Can you work these out from the model? Positions are in its coordinate system, mm. Coordinates: 2 decimals unless noted, no trailing zeros. Loops run counter-clockwise (first coordinate to the right, second up) from the corner with the lowest first, then second, coordinate; pieces in that order, holes last. Notation, with made-up numbers: (52.25, 26) -> (69.25, 26) arc R27 cw to (69.25, 56) -> close; hole circle Ø4 at (55, 74.5). An arc over 180 degrees is marked (long way). Put each result on its own line as item: value. Start each with the question number.
Item 1: Please list where these lines run through material, in increasing order: L1, parallel to Y at x = 298.65, z = 25.27; L2, parallel to X at y = 3, z = 12; L3, parallel to X at y = 31.5, z = 26. Write a range as from..to.
Item 2: If we section it at A-A on x = 29.5: Please give me the cut outline in (y, z), plus the area to 3 significant figures.
Item 3: Will these pins go through, and if not, where does the flat tip stop? P1, Ø6, axis at x = 187, z = 31, coming from the +Y side; P2, Ø5, axis at x = 217.5, z = 27.5, coming from the +Y side; P3, Ø3.5, axis at y = 27.39, z = 25.27, coming from the +X side.
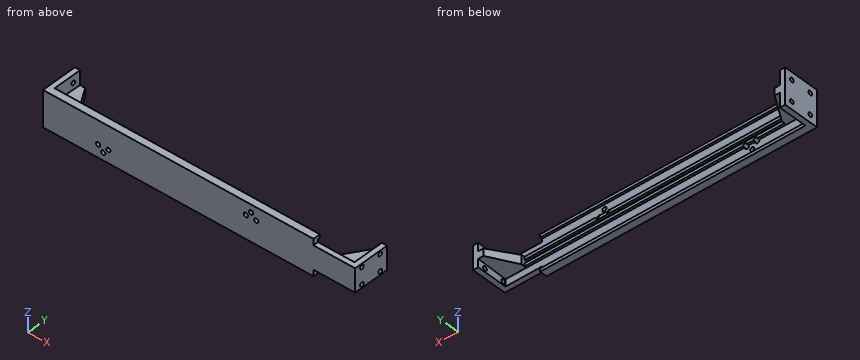
```python
from build123d import *

# Parameters (mm, degrees)
EXTRUDE_1_DEPTH          = 34.54
CUT_EXTRUDE_1_REACH      = 305.978
SKETCH_2_W               = 40
SKETCH_2_H               = 6
SKETCH_3_R               = 2
CUT_EXTRUDE_2_DEPTH      = 5
SKETCH_4_R               = 2
CUT_EXTRUDE_3_DEPTH      = 5
RIB_START                = 5
RIB_7_DEPTH              = 20
RIB_START_2              = 12.730059485
RIB_7_2_DEPTH            = 9.07988103
RIB_START_3              = 275
RIB_19_DEPTH             = 20
RIB_START_4              = 147.269934089
RIB_19_2_DEPTH           = 35.576868781
EXTRUDE_2_REACH          = 301.045
SKETCH_8_W               = 3
SKETCH_8_H               = 2
CUT_EXTRUDE_4_DEPTH      = 304.978058419
CUT_EXTRUDE_4_DEPTH_BACK = 304.978058419
SKETCH_9_W               = 35
SKETCH_9_H               = 3
CUT_EXTRUDE_5_REACH      = 305.978
SKETCH_10_R              = 2
CUT_EXTRUDE_6_REACH      = 305.978
SKETCH_11_R              = 2


with BuildPart() as part:
    # 草图1 → 凸台-拉伸1 (new body)
    with BuildSketch(Plane.XY):
        Polygon((0, 0), (300, 0), (300, 34.78), (295, 34.78), (295, 5), (5, 5), (5, 34.78), (0, 34.78), align=None)
    extrude(amount=EXTRUDE_1_DEPTH)

    # 切除-拉伸1: up to this face of the body (flat: up to its plane)
    cut_extrude_1_end = Plane(part.part.faces().sort_by_distance((297.5, 34.78, 17.27))[0])
    # 草图2 → 切除-拉伸1 (cut, up to the picked face)
    with BuildSketch(Plane.XZ, mode=Mode.PRIVATE) as cut_extrude_1_sk1:
        with Locations((280, 31.54)):
            Rectangle(SKETCH_2_W, SKETCH_2_H)
    cut_extrude_1_tool1 = split(extrude(cut_extrude_1_sk1.sketch, amount=-CUT_EXTRUDE_1_REACH, mode=Mode.PRIVATE), bisect_by=cut_extrude_1_end, keep=Keep.BOTH, mode=Mode.PRIVATE)
    # 草图2 → 切除-拉伸1 (cut, up to the picked face)
    with BuildSketch(Plane.XZ, mode=Mode.PRIVATE) as cut_extrude_1_sk2:
        with Locations((280, 3)):
            Rectangle(SKETCH_2_W, SKETCH_2_H)
    cut_extrude_1_tool2 = split(extrude(cut_extrude_1_sk2.sketch, amount=-CUT_EXTRUDE_1_REACH, mode=Mode.PRIVATE), bisect_by=cut_extrude_1_end, keep=Keep.BOTH, mode=Mode.PRIVATE)
    add(cut_extrude_1_tool1.solids().sort_by(Axis((280, 0, 31.54), (0, 1, 0)))[0], mode=Mode.SUBTRACT)
    add(cut_extrude_1_tool2.solids().sort_by(Axis((280, 0, 3), (0, 1, 0)))[0], mode=Mode.SUBTRACT)

    # 草图3 → 切除-拉伸2 (cut)
    with BuildSketch(Plane(origin=(300, 0, 0), x_dir=(0, 0, -1), z_dir=(1, 0, 0))):
        with Locations((-25.27, 7.39)):
            Circle(SKETCH_3_R)
        with Locations((-25.27, 27.39)):
            Circle(SKETCH_3_R)
        with Locations((-9.27, 27.39)):
            Circle(SKETCH_3_R)
        with Locations((-9.27, 7.39)):
            Circle(SKETCH_3_R)
    extrude(amount=-CUT_EXTRUDE_2_DEPTH, mode=Mode.SUBTRACT)

    # 草图4 → 切除-拉伸3 (cut)
    with BuildSketch(Plane.ZY):
        with Locations(Location((7.27, 27.39, 0), (0, 0, 270))):
            Circle(SKETCH_4_R)
        with Locations(Location((27.27, 27.39, 0), (0, 0, 270))):
            Circle(SKETCH_4_R)
        with Locations(Location((27.27, 7.39, 0), (0, 0, 270))):
            Circle(SKETCH_4_R)
        with Locations(Location((7.27, 7.39, 0), (0, 0, 270))):
            Circle(SKETCH_4_R)
    extrude(amount=-CUT_EXTRUDE_3_DEPTH, mode=Mode.SUBTRACT)

    # 筋7: read off the stored shape, not the designer's step
    # 筋7 outline → 筋7 (add)
    with BuildSketch(Plane.YZ.offset(RIB_START)):
        Polygon((34.78, 13.77), (34.78, 20.77), (5, 21.809940515), (5, 12.730059485), align=None)
    extrude(amount=RIB_7_DEPTH)

    # Rib 7 2 outline → Rib 7 2 (cut)
    with BuildSketch(Plane.XY.offset(RIB_START_2)):
        Polygon((25, 34.78), (10, 34.78), (25, 10), align=None)
    extrude(amount=RIB_7_2_DEPTH, mode=Mode.SUBTRACT)

    # 筋19: read off the stored shape, not the designer's step
    # 筋19 outline → 筋19 (add)
    with BuildSketch(Plane.YZ.offset(RIB_START_3)):
        Polygon((34.78, 13.77), (34.78, 20.77), (5, 21.809940515), (5, 12.730059485), align=None)
    extrude(amount=RIB_19_DEPTH)

    # Rib 19 2 outline → Rib 19 2 (cut)
    with BuildSketch(Plane(origin=(0, 0, 0), x_dir=(0.8556156704777578, -0.5172963390397041, -0.018064386206466228), z_dir=(0.5176116540736858, 0.8550944525297293, 0.02986055625713262)).offset(RIB_START_4)):
        Polygon((229.730516914, -21.273162039), (229.888231169, -12.547807193), (216, -12.547807193), (216, -23), (229.699303632, -23), align=None)
    extrude(amount=RIB_19_2_DEPTH, mode=Mode.SUBTRACT)

    # 凸台-拉伸2: up to this face of the body (flat: up to its plane)
    extrude_2_end = Plane(part.part.faces().sort_by_distance((295, 20.622218635, 24.86118076))[0])
    # 草图8 → 凸台-拉伸2 (add, up to the picked face)
    with BuildSketch(Plane(origin=(5, 0, 0), x_dir=(0, 0, -1), z_dir=(1, 0, 0)), mode=Mode.PRIVATE) as extrude_2_sk1:
        with Locations((-33.04, 6)):
            Rectangle(SKETCH_8_W, SKETCH_8_H)
    extrude_2_tool1 = split(extrude(extrude_2_sk1.sketch, amount=EXTRUDE_2_REACH, mode=Mode.PRIVATE), bisect_by=extrude_2_end, keep=Keep.BOTH, mode=Mode.PRIVATE)
    # 草图8 → 凸台-拉伸2 (add, up to the picked face)
    with BuildSketch(Plane(origin=(5, 0, 0), x_dir=(0, 0, -1), z_dir=(1, 0, 0)), mode=Mode.PRIVATE) as extrude_2_sk2:
        Polygon((-21.740098976, 7), (-21.809940515, 5), (-18.740098976, 5), (-18.740098976, 7), align=None)
    extrude_2_tool2 = split(extrude(extrude_2_sk2.sketch, amount=EXTRUDE_2_REACH, mode=Mode.PRIVATE), bisect_by=extrude_2_end, keep=Keep.BOTH, mode=Mode.PRIVATE)
    # 草图8 → 凸台-拉伸2 (add, up to the picked face)
    with BuildSketch(Plane(origin=(5, 0, 0), x_dir=(0, 0, -1), z_dir=(1, 0, 0)), mode=Mode.PRIVATE) as extrude_2_sk3:
        Polygon((-15.799901024, 7), (-15.799901024, 5), (-12.730059485, 5), (-12.799901024, 7), align=None)
    extrude_2_tool3 = split(extrude(extrude_2_sk3.sketch, amount=EXTRUDE_2_REACH, mode=Mode.PRIVATE), bisect_by=extrude_2_end, keep=Keep.BOTH, mode=Mode.PRIVATE)
    # 草图8 → 凸台-拉伸2 (add, up to the picked face)
    with BuildSketch(Plane(origin=(5, 0, 0), x_dir=(0, 0, -1), z_dir=(1, 0, 0)), mode=Mode.PRIVATE) as extrude_2_sk4:
        with Locations((-1.5, 6)):
            Rectangle(SKETCH_8_W, SKETCH_8_H)
    extrude_2_tool4 = split(extrude(extrude_2_sk4.sketch, amount=EXTRUDE_2_REACH, mode=Mode.PRIVATE), bisect_by=extrude_2_end, keep=Keep.BOTH, mode=Mode.PRIVATE)
    add(extrude_2_tool1.solids().sort_by(Axis((5, 6, 33.04), (1, 0, 0)))[0])
    add(extrude_2_tool2.solids().sort_by(Axis((5, 5.996165, 20.257626), (1, 0, 0)))[0])
    add(extrude_2_tool3.solids().sort_by(Axis((5, 5.996165, 14.282374), (1, 0, 0)))[0])
    add(extrude_2_tool4.solids().sort_by(Axis((5, 6, 1.5), (1, 0, 0)))[0])

    # 草图9 → 切除-拉伸4 (cut, two sides: drawn at the far end of the back side and taken through both)
    with BuildSketch(Plane.XZ.offset(-CUT_EXTRUDE_4_DEPTH_BACK)):
        with Locations((277.5, 1.5)):
            Rectangle(SKETCH_9_W, SKETCH_9_H)
        with Locations((277.5, 33.04)):
            Rectangle(SKETCH_9_W, SKETCH_9_H)
    extrude(amount=CUT_EXTRUDE_4_DEPTH + CUT_EXTRUDE_4_DEPTH_BACK, mode=Mode.SUBTRACT)

    # 切除-拉伸5: up to this face of the body (flat: up to its plane)
    cut_extrude_5_end = Plane(part.part.faces().sort_by_distance((132.5, 7, 33.04))[0])
    # 草图10 → 切除-拉伸5 (cut, up to the picked face)
    with BuildSketch(Plane.XZ, mode=Mode.PRIVATE) as cut_extrude_5_sk1:
        with Locations(Location((205, 22.27, 0), (0, 0, 270))):
            Circle(SKETCH_10_R)
    cut_extrude_5_tool1 = split(extrude(cut_extrude_5_sk1.sketch, amount=-CUT_EXTRUDE_5_REACH, mode=Mode.PRIVATE), bisect_by=cut_extrude_5_end, keep=Keep.BOTH, mode=Mode.PRIVATE)
    # 草图10 → 切除-拉伸5 (cut, up to the picked face)
    with BuildSketch(Plane.XZ, mode=Mode.PRIVATE) as cut_extrude_5_sk2:
        with Locations(Location((200, 27.27, 0), (0, 0, 270))):
            Circle(SKETCH_10_R)
    cut_extrude_5_tool2 = split(extrude(cut_extrude_5_sk2.sketch, amount=-CUT_EXTRUDE_5_REACH, mode=Mode.PRIVATE), bisect_by=cut_extrude_5_end, keep=Keep.BOTH, mode=Mode.PRIVATE)
    # 草图10 → 切除-拉伸5 (cut, up to the picked face)
    with BuildSketch(Plane.XZ, mode=Mode.PRIVATE) as cut_extrude_5_sk3:
        with Locations(Location((195, 22.27, 0), (0, 0, 270))):
            Circle(SKETCH_10_R)
    cut_extrude_5_tool3 = split(extrude(cut_extrude_5_sk3.sketch, amount=-CUT_EXTRUDE_5_REACH, mode=Mode.PRIVATE), bisect_by=cut_extrude_5_end, keep=Keep.BOTH, mode=Mode.PRIVATE)
    add(cut_extrude_5_tool1.solids().sort_by(Axis((205, 0, 22.27), (0, 1, 0)))[0], mode=Mode.SUBTRACT)
    add(cut_extrude_5_tool2.solids().sort_by(Axis((200, 0, 27.27), (0, 1, 0)))[0], mode=Mode.SUBTRACT)
    add(cut_extrude_5_tool3.solids().sort_by(Axis((195, 0, 22.27), (0, 1, 0)))[0], mode=Mode.SUBTRACT)

    # 切除-拉伸6: up to this face of the body (flat: up to its plane)
    cut_extrude_6_end = Plane(part.part.faces().sort_by_distance((150, 7, 14.299901024))[0])
    # 草图11 → 切除-拉伸6 (cut, up to the picked face)
    with BuildSketch(Plane.XZ, mode=Mode.PRIVATE) as cut_extrude_6_sk1:
        with Locations(Location((52.9, 12.27, 0), (0, 0, 270))):
            Circle(SKETCH_11_R)
    cut_extrude_6_tool1 = split(extrude(cut_extrude_6_sk1.sketch, amount=-CUT_EXTRUDE_6_REACH, mode=Mode.PRIVATE), bisect_by=cut_extrude_6_end, keep=Keep.BOTH, mode=Mode.PRIVATE)
    # 草图11 → 切除-拉伸6 (cut, up to the picked face)
    with BuildSketch(Plane.XZ, mode=Mode.PRIVATE) as cut_extrude_6_sk2:
        with Locations(Location((62.9, 12.27, 0), (0, 0, 270))):
            Circle(SKETCH_11_R)
    cut_extrude_6_tool2 = split(extrude(cut_extrude_6_sk2.sketch, amount=-CUT_EXTRUDE_6_REACH, mode=Mode.PRIVATE), bisect_by=cut_extrude_6_end, keep=Keep.BOTH, mode=Mode.PRIVATE)
    # 草图11 → 切除-拉伸6 (cut, up to the picked face)
    with BuildSketch(Plane.XZ, mode=Mode.PRIVATE) as cut_extrude_6_sk3:
        with Locations(Location((57.9, 7.27, 0), (0, 0, 270))):
            Circle(SKETCH_11_R)
    cut_extrude_6_tool3 = split(extrude(cut_extrude_6_sk3.sketch, amount=-CUT_EXTRUDE_6_REACH, mode=Mode.PRIVATE), bisect_by=cut_extrude_6_end, keep=Keep.BOTH, mode=Mode.PRIVATE)
    add(cut_extrude_6_tool1.solids().sort_by(Axis((52.9, 0, 12.27), (0, 1, 0)))[0], mode=Mode.SUBTRACT)
    add(cut_extrude_6_tool2.solids().sort_by(Axis((62.9, 0, 12.27), (0, 1, 0)))[0], mode=Mode.SUBTRACT)
    add(cut_extrude_6_tool3.solids().sort_by(Axis((57.9, 0, 7.27), (0, 1, 0)))[0], mode=Mode.SUBTRACT)


solid = part.part
```
Solutions:
1. L1: 0..5.39, 9.39..25.39, 29.39..34.78
1. L2: 0..50.92, 54.88..60.92, 64.88..300
1. L3: 0..5, 295..300
2. outline: (0, 0) -> (7, 0) -> (7, 3) -> (5, 3) -> (5, 12.73) -> (7, 12.8) -> (7, 15.8) -> (5, 15.8) -> (5, 18.74) -> (7, 18.74) -> (7, 21.74) -> (5, 21.81) -> (5, 31.54) -> (7, 31.54) -> (7, 34.54) -> (0, 34.54) -> close
2. area: 197 mm^2
3. P1: y = 7
3. P2: y = 5
3. P3: x = 5
